Work out the finished part from the listing and answer in its coordinate system (mm). Coordinates: 2 decimals unless noted, no trailing zeros. Order: outer loops, then holes, each group sorted by start corner. A loop starts at its lowest first (then second) coordinate and runs counter-clockwise, first axis right, second up. Notation, with made-up numbers: M 35.25,50.25 L 71.25,50.25 A21 ccw 71.25,67.25 Z; hole C 35.5,53.25 d11. An arc over 180 degrees is marked long. Use a Markdown table: item, result.
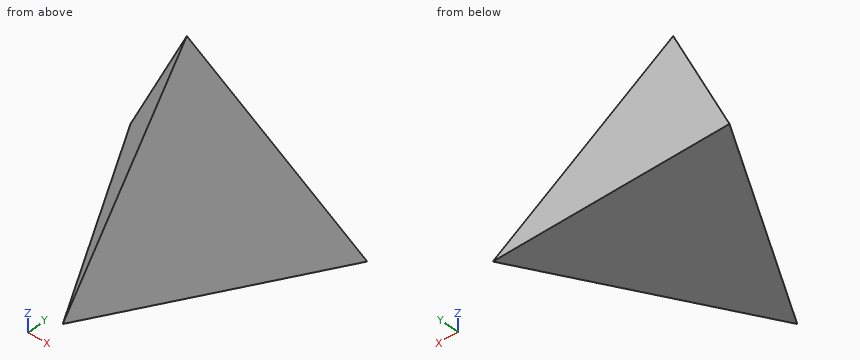
Solid Edge part; units mm, degrees
sketch "Sketch1" plane through (0, 0, 0) normal (0, 0, 1) x (1, 0, 0)
  line L0 (-15, 8.6603) -> (0, -17.3205)
  line L1 (0, -17.3205) -> (15, 8.6603)
  line L2 (15, 8.6603) -> (-15, 8.6603)
extrude "Protrusion1" add sketch "Sketch1" along normal up to vertex (24.4949 mm away)
sketch "Sketch2" plane through (0, 0, 0) normal (1, 0, 0) x (0, 1, 0)
  line L0 (8.6603, 24.4949) -> (0, 24.4949)
  line L1 (0, 24.4949) -> (8.6603, 0)
  line L2 (8.6603, 0) -> (8.6603, 24.4949)
extrude "Cutout1" cut sketch "Sketch2" along normal mid plane 30
pattern_circular "Pattern1" count 3 over 360 about axis through (0, 0, 24.4949) along (0, 0, 1) of "Cutout1"
1. Section C-C on z = 17 is taken. Determine the outline of the cut face in (x, y), then the cut area to 3 significant figures.
Answers below:
| item | result |
|---|---|
| outline | M -4.59,2.65 L 0,-5.3 L 4.59,2.65 Z |
| area | 36.5 mm² |
2. Flat-ended cylindrical pins translate along their axes: P1, Ø8, axis at x = -12, z = 6.5, coming from the -Y side; P2, Ø8, axis at y = 3.5, z = 7, coming from the +X side; P3, Ø5, axis at x = -2, z = 8.5, coming from the -Y side. Find the tip coordinate at first contact, or state that the pin passes through.
Answers below:
| item | result |
|---|---|
| P1 | y = 0.58 |
| P2 | x = 11.99 |
| P3 | y = -12.37 |
3. Find the intervals of material crossed by probe 1 along Z at (x, y) = (6.5, 2); probe 2 along Z at (x, y) = (-1.5, -9); probe 3 along Y at (x, z) = (3.5, 1.5), in increasing order.
Answers below:
| item | result |
|---|---|
| probe 1 | 0 to 11.4 |
| probe 2 | 0 to 8.09 |
| probe 3 | -10.2 to 8.13 |
